Part model, mm, in its own coordinate system. A direction names the side the tool comes from. Coordinates: 2 decimals unless noted, no trailing zeros. Order: outer loops, then holes, each group sorted by start corner. A loop starts at its lowest first (then second) coordinate and runs counter-clockwise, first axis right, second up.
```python
from build123d import *

# Parameters (mm, degrees)
SKETCH_1_R      = 10
EXTRUDE_1_DEPTH = 70


with BuildPart() as part:
    # Эскиз1 → Бобышка-Вытянуть1 (new body)
    with BuildSketch(Plane(origin=(0, 0, 0), x_dir=(1, 0, 0), z_dir=(0, 1, 0))):
        with Locations(Location((0, 0, 0), (0, 0, 270))):
            Circle(SKETCH_1_R)
    extrude_1 = extrude(amount=EXTRUDE_1_DEPTH)

    # Эскиз4 → Отверстие с зазором M41 (revolve, cut)
    with BuildSketch(Plane(origin=(0, 70, 0), x_dir=(0, 0, 1), z_dir=(1, 0, 0))):
        Polygon((0, 0), (0, 17.351936393), (2.25, 16), (2.25, 0), align=None)
    hole_wizard_m41 = revolve(axis=Axis((0, 76.35, 0), (0, -1, 0)), mode=Mode.SUBTRACT)

    # Зеркальное отражение1: Бобышка-Вытянуть1, Отверстие с зазором M41 across plane
    add(extrude_1.mirror(Plane.ZX))
    add(hole_wizard_m41.mirror(Plane.ZX), mode=Mode.SUBTRACT)


solid = part.part
```
(1) Probe line 1 (X direction, y = 66.25, z = 0); line 2 (X direction, y = -47, z = 0); line 3 (Z direction, x = 8.75, y = -39.5). List the from-to ranges inside material, lowest first.
(2) Pull direction Z, two halves, no side cores. Call faces 1 (the face through (-0.12, 52.88, 0.37)), 2 (the face through (-9.76, 0.98, -2.17)), 3 (the face through (2.4, -70, -0.1)): +Z half, -Z half, draft (parallel to the pull), parting line (faces both ways), or undercut.
(3) Tool access for faces 4 (the face through (-2.23, 62.11, -0.29)), 5 (the face through (-2.23, -62.11, -0.29)), 6 (the face through (2.4, 70, -0.1)): list every direction of +Z, -Z, +X, -X, +Y, -Y with a clear straight run to the whole face (end or side of a thin tool).
(4) Slice it at B-B, the plane x = 3.5. Give the cut face in (y, z), then the cut area to 3 significant figures.
(5) Slice it at A-A, the plane y = 20.5. Give the cut face in (x, z), then the cut area to 3 significant figures.
(6) Slice it at C-C, the plane z = -7.75. Give the cut face in (x, y).
(7) Drop flat-ended pins along their axis: pin 1 (2 mm diameter, centred on x = 1.5, z = 1, fed in from +Y); pin 2 (2.5 mm diameter, centred on x = 0, z = 0, fed in from +Y); pin 3 (2 mm diameter, centred on x = 3, y = 24, fed in from +Z); pin 4 (8 mm diameter, centred on y = 10.5, z = -6.5, fed in from +X). Give the stop position or say it passes through.
Here are the results:
1. line 1: x = -10 to -2.25, 2.25 to 10
1. line 2: x = -10 to 10
1. line 3: z = -4.84 to 4.84
2. face 1: undercut
2. face 2: parting line
2. face 3: draft
3. face 4: +Y
3. face 5: -Y
3. face 6: +Z, -Z, +X, -X, +Y
4. outline: (-70, -9.37) - (70, -9.37) - (70, 9.37) - (-70, 9.37) - close
4. area: 2,620 mm2
5. outline: circle Ø20 at (0, 0)
5. area: 314 mm2
6. outline: (-6.32, -70) - (6.32, -70) - (6.32, 70) - (-6.32, 70) - close
7. pin 1: stops at y = 70
7. pin 2: stops at y = 53.4
7. pin 3: stops at z = 9.8
7. pin 4: stops at x = 9.68
